Read the model definition and answer for the solid it produces. Units are mm, in the model's axes. Face numbers are marked on the shaded views. A direction names the side the tool comes from. Round coordinates to 2 decimals unless told otherwise and drop trailing zeros. Order: outer loops, then holes, each group sorted by start corner. A loop starts at its lowest first (then second) coordinate and runs counter-clockwise, first axis right, second up. Notation, with made-up numbers: (0, -15) - (55, -15) arc R19 cw to (55, 18) - close; hole circle Ø6 at (50.5, 80.25). An arc over 180 degrees is marked (long way). One line per question, with ' | ' between items. Start each with the question number.
1) The part is cut by section D-D, the plane z = 1.75. Give the vertices of the cut face in (x, y).
2) The part is cut by section C-C, the plane y = 1.5. Give the vertices of the cut face in (x, z).
3) Flat-ended cylindrical pins translate along their axes: pin 1 (0.5 mm diameter, centred on x = 46, y = 11.5, fed in from +Z); pin 2 (0.8 mm diameter, centred on x = 14, y = 27.5, fed in from -Z); pin 3 (10 mm diameter, centred on x = 23.5, y = 13.5, fed in from +Z); pin 4 (1 mm diameter, centred on x = 13, y = 9.5, fed in from +Z). Find the tip coordinate at first contact, or state that the pin passes through.
4) The part is cut by section A-A, the plane z = 6.5. Give the vertices of the cut face in (x, y), plus the area to 4 significant figures.
5) Straight lines are drawn through the part: line 1 (X direction, y = -6.5, z = 1); line 2 (X direction, y = -4, z = 8); line 3 (Y direction, x = 30.5, z = 7). For each, find the intervals that lie inside material, in ascending order. Write a range as from..to.
6) The part is cut by section B-B, the plane x = 14.5. Give the vertices of the cut face in (y, z), plus the area to 4 significant figures.
7) The mould has two halves that part along Y. Classify the marked faces 3, 4, 5 and 6: pulls with the +Y half, pulls with the -Y half, needs draft (parallel to the pull), parting line crosses it, or undercut.
8) For the marked faces 1 and 2, determine the directions among +Z, -Z, +X, -X, +Y, -Y from which every point of the face is accessible in a straight line to the end or side of a thin tool.
from build123d import *

# Parameters (mm, degrees)
CROQUIS1_W              = 96.5
CROQUIS1_H              = 34.25
SALIENTE_EXTRUIR1_DEPTH = 0.75
CROQUIS3_W              = 98.5
CROQUIS3_H              = 36.25
CROQUIS3_W_2            = 96.5
CROQUIS3_H_2            = 34.25
SALIENTE_EXTRUIR2_DEPTH = 11.75
SALIENTE_EXTRUIR3_DEPTH = 4.75
SALIENTE_EXTRUIR4_DEPTH = 3
SALIENTE_EXTRUIR5_DEPTH = 2.5
CROQUIS8_W              = 1
CROQUIS8_H              = 14.1
CORTAR_EXTRUIR1_DEPTH   = 2.5
CORTAR_EXTRUIR2_DEPTH   = 2.5
CORTAR_EXTRUIR3_DEPTH   = 1.5
CROQUIS11_W             = 7
CROQUIS11_H             = 3.2
CORTAR_EXTRUIR4_DEPTH   = 10


with BuildPart() as part:
    # Croquis1 → Saliente-Extruir1 (new body)
    with BuildSketch(Plane.XY):
        with Locations((-2.825600583, 9.945957096)):
            Rectangle(CROQUIS1_W, CROQUIS1_H)
    extrude(amount=SALIENTE_EXTRUIR1_DEPTH)

    # Croquis3 → Saliente-Extruir2 (add)
    with BuildSketch(Plane(origin=(0, 0, 0), x_dir=(-1, 0, 0), z_dir=(0, 0, -1))):
        with Locations((2.825600583, 9.945957096)):
            Rectangle(CROQUIS3_W, CROQUIS3_H)
        with Locations((2.825600583, 9.945957096)):
            Rectangle(CROQUIS3_W_2, CROQUIS3_H_2, mode=Mode.SUBTRACT)
    extrude(amount=-SALIENTE_EXTRUIR2_DEPTH)

    # Croquis5 → Saliente-Extruir3 (add)
    with BuildSketch(Plane.XY.offset(0.75)):
        Polygon((-5.725600583, -7.179042904), (-5.725600583, 17.120957096), (45.424399417, 17.120957096), (45.424399417, 27.070957096), (-6.725600583, 27.070957096), (-6.725600583, -7.179042904), align=None)
    extrude(amount=SALIENTE_EXTRUIR3_DEPTH)

    # Croquis6 → Saliente-Extruir4 (add)
    with BuildSketch(Plane.XY):
        Polygon((-6.725600583, 9.220957096), (-6.725600583, 27.070957096), (-51.075600583, 27.070957096), (-51.075600583, -7.179042904), (-45.525600583, -7.179042904), (-45.525600583, 9.220957096), align=None)
    extrude(amount=SALIENTE_EXTRUIR4_DEPTH)

    # Croquis7 → Saliente-Extruir5 (add)
    with BuildSketch(Plane.XY.offset(3)):
        Polygon((-34.125600583, 27.070957096), (-51.075600583, 27.070957096), (-51.075600583, -7.179042904), (-45.525600583, -7.179042904), (-45.525600583, 9.220957096), (-6.725600583, 9.220957096), (-6.725600583, 12.970957096), (-34.125600583, 12.970957096), align=None)
    extrude(amount=SALIENTE_EXTRUIR5_DEPTH)

    # Croquis8 → Cortar-Extruir1 (cut)
    with BuildSketch(Plane.XY.offset(5.5)):
        with Locations((-6.225600583, 20.020957096)):
            Rectangle(CROQUIS8_W, CROQUIS8_H)
    extrude(amount=-CORTAR_EXTRUIR1_DEPTH, mode=Mode.SUBTRACT)

    # Croquis9 → Cortar-Extruir2 (cut)
    with BuildSketch(Plane.XZ.offset(-27.070957096)):
        Polygon((10.224399417, 10.98), (17.624399417, 10.98), (17.624399417, 8.98), (16.624399417, 7.98), (11.224399417, 7.98), (10.224399417, 8.98), align=None)
        with BuildLine():
            Line((33.524399417, 11.18), (39.524399417, 11.18))
            ThreePointArc((39.524399417, 11.18), (41.124399417, 9.58), (39.524399417, 7.98))
            Line((39.524399417, 7.98), (33.524399417, 7.98))
            ThreePointArc((33.524399417, 7.98), (31.924399417, 9.58), (33.524399417, 11.18))
        make_face()
    extrude(amount=-CORTAR_EXTRUIR2_DEPTH, mode=Mode.SUBTRACT)

    # Croquis10 → Cortar-Extruir3 (cut)
    with BuildSketch(Plane.XY.offset(11.75)):
        Polygon((-7.825600583, 36.220855399), (2.174399417, 36.220855399), (2.174399417, 14.945957096), (54.759857348, 14.945957096), (54.759857348, 4.945957096), (2.174399417, 4.945957096), (2.174399417, -27.159073942), (-7.825600583, -27.159073942), (-7.825600583, 4.945957096), (-73.50393186, 4.945957096), (-73.50393186, 14.945957096), (-7.825600583, 14.945957096), align=None)
    extrude(amount=-CORTAR_EXTRUIR3_DEPTH, mode=Mode.SUBTRACT)

    # Croquis11 → Cortar-Extruir4 (cut)
    with BuildSketch(Plane.XZ.offset(8.179042904)):
        with Locations((36.924399417, 10.15)):
            Rectangle(CROQUIS11_W, CROQUIS11_H)
    extrude(amount=-CORTAR_EXTRUIR4_DEPTH, mode=Mode.SUBTRACT)


solid = part.part
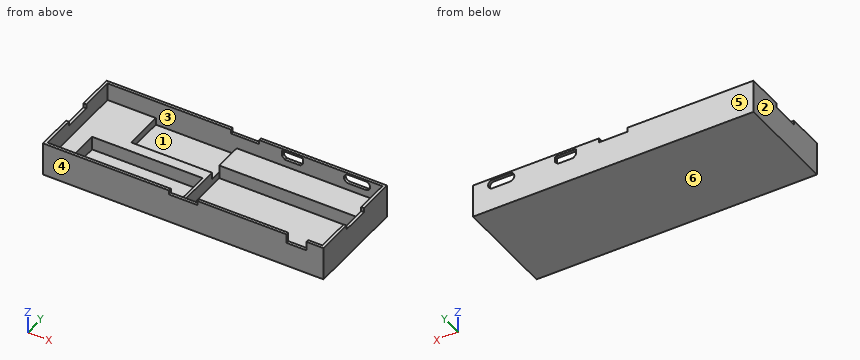
Values:
1) outline: (-52.08, -8.18) - (46.42, -8.18) - (46.42, 28.07) - (-52.08, 28.07) - close; hole (-45.53, -7.18) - (-6.73, -7.18) - (-6.73, 9.22) - (-45.53, 9.22) - close; hole (-5.73, -7.18) - (45.42, -7.18) - (45.42, 17.12) - (-5.73, 17.12) - close
2) outline: (-52.08, 0) - (46.42, 0) - (46.42, 11.75) - (45.42, 11.75) - (45.42, 0.75) - (-5.73, 0.75) - (-5.73, 5.5) - (-6.73, 5.5) - (-6.73, 0.75) - (-45.53, 0.75) - (-45.53, 5.5) - (-51.08, 5.5) - (-51.08, 11.75) - (-52.08, 11.75) - close
3) pin 1: stops at z = 10.25 | pin 2: stops at z = 0 | pin 3: stops at z = 5.5 | pin 4: stops at z = 0.75
4) outline: (-52.08, -8.18) - (46.42, -8.18) - (46.42, 28.07) - (-52.08, 28.07) - close; hole (-51.08, -7.18) - (45.42, -7.18) - (45.42, 27.07) - (-51.08, 27.07) - close | area: 265.5 mm^2
5) line 1: x = -52.08..-45.53, -6.73..-5.73, 45.42..46.42 | line 2: x = -52.08..-51.08, 45.42..46.42 | line 3: y = -8.18..-7.18, 27.07..28.07
6) outline: (-8.18, 0) - (28.07, 0) - (28.07, 7.98) - (27.07, 7.98) - (27.07, 5.5) - (17.12, 5.5) - (17.12, 0.75) - (-7.18, 0.75) - (-7.18, 11.75) - (-8.18, 11.75) - close; (27.07, 10.98) - (28.07, 10.98) - (28.07, 11.75) - (27.07, 11.75) - close | area: 93.45 mm^2
7) face 3: undercut | face 4: pulls with the -Y half | face 5: pulls with the +Y half | face 6: needs draft
8) face 1: +Z | face 2: +Z, -Z, -X, +Y, -Y
